For this review, take the finished solid that the model builds, in its own axes (mm). Face numbers are marked on the shaded views. Round coordinates to 2 decimals unless told otherwise and drop trailing zeros. Order: outer loops, then holes, each group sorted by start corner. A loop starts at its lowest first (then second) coordinate and runs counter-clockwise, first axis right, second up.
Autodesk Inventor part; units mm, degrees
ref_plane "YZ Plane" through (0, 0, 0) normal (1, 0, 0) x (0, 1, 0)
ref_plane "XZ Plane" through (0, 0, 0) normal (0, 1, 0) x (-1, 0, 0)
ref_plane "XY Plane" through (0, 0, 0) normal (0, 0, 1) x (1, 0, 0)
sketch "Sketch1" plane through (0, 0, 0) normal (0, 1, 0) x (-1, 0, 0)
  line L0 (0, 0) -> (0, -25.4)
  line L1 (0, -25.4) -> (558.8, -25.4)
  line L2 (558.8, -25.4) -> (558.8, 0)
  line L3 (558.8, 0) -> (0, 0)
  dimension "d0" = 25.4
  dimension "d1" = 558.8
extrude "Plate1" add sketch "Sketch1" along normal blind 0.9652
sketch "Sketch2" plane through (-558.8, 0.1746, -0.5536) normal (0, 0.819152, 0.5735764) x (-1, 0, 0)
  line L0 (-558.8, 0) -> (0, 0)
  line L1 (0, 0) -> (0, 31.75)
  line L2 (0, 31.75) -> (-558.8, 31.75)
  line L3 (-558.8, 31.75) -> (-558.8, 0)
edge flange "Flange1" height 31.75 angle 35 thickness 0.9652 bend radius 0.9652 thickness toward (0, 0.819152, 0.5735764) relief tear relief width 0.9652 relief depth 0.4826 edges at (-279.4, 0, 0) wall of the first edge with corners at (0, 0.1746, -0.5536) (-558.8, 0.1746, -0.5536) (-558.8, -18.0365, 25.4545) (0, -18.0365, 25.4545)
bend "Bend1"
corner "Corner1"
sketch "Sketch3" plane through (0, -17.2459, 24.9008) normal (0, -0.819152, 0.5735764) x (1, 0, 0)
  line L0 (-558.8, 0) -> (0, 0)
  line L1 (0, 0) -> (0, 31.75)
  line L2 (0, 31.75) -> (-558.8, 31.75)
  line L3 (-558.8, 31.75) -> (-558.8, 0)
edge flange "Flange2" height 31.75 angle 70 thickness 0.9652 bend radius 0.9652 thickness toward (0, -0.819152, 0.5735764) relief tear relief width 0.9652 relief depth 0.4826 edges at (-279.4, -17.2459, 26.0081) wall of the first edge with corners at (-558.8, -17.2459, 24.9008) (0, -17.2459, 24.9008) (0, 0.9652, 50.9089) (-558.8, 0.9652, 50.9089)
bend "Bend2"
corner "Corner2"
sketch "Sketch4" plane through (-558.8, 0, 50.9089) normal (0, 1, 0) x (-1, 0, 0)
  line L0 (-558.8, 0) -> (0, 0)
  line L1 (0, 0) -> (0, 25.4)
  line L2 (0, 25.4) -> (-558.8, 25.4)
  line L3 (-558.8, 25.4) -> (-558.8, 0)
edge flange "Flange3" height 25.4 angle 35 thickness 0.9652 bend radius 0.9652 thickness toward (0, 1, 0) relief tear relief width 0.9652 relief depth 0.4826 edges at (-279.4, 0.1746, 51.4625) wall of the first edge with corners at (0, 0, 50.9089) (-558.8, 0, 50.9089) (-558.8, 0, 76.3089) (0, 0, 76.3089)
bend "Bend3"
corner "Corner3"
sketch "Sketch5" plane through (0, 0.9652, 0) normal (0, 1, 0) x (1, 0, 0)
  line L0 (0, -51.5176) -> (-25.4, -51.5176)
  line L1 (0, -51.5176) -> (0, -50.4103)
  line L2 (0, -51.5176) -> (0, 0.6087)
  line L3 (0, 0.6087) -> (-25.4, 0.6087)
  line L4 (-25.4, 0.6087) -> (-25.4, -51.5176)
  line L5 (-114.3, -65.0679) -> (-88.9, -65.0679) construction
  line L6 (-114.3, -67.6079) -> (-88.9, -67.6079)
  line L7 (-88.9, -62.5279) -> (-114.3, -62.5279)
  arc A0 (-114.3, -62.5279) -> (-114.3, -67.6079) centre (-114.3, -65.0679) ccw
  arc A1 (-88.9, -67.6079) -> (-88.9, -62.5279) centre (-88.9, -65.0679) ccw
  line L8 (-87.7062, -24.2598) -> (31.8104, -24.2598) construction
  line L9 (-114.3, 19.0882) -> (-88.9, 19.0882)
  line L10 (-88.9, 14.0082) -> (-114.3, 14.0082)
  arc A2 (-114.3, 19.0882) -> (-114.3, 14.0082) centre (-114.3, 16.5482) ccw
  arc A3 (-88.9, 14.0082) -> (-88.9, 19.0882) centre (-88.9, 16.5482) ccw
  line L11 (0, -76.3089) -> (-558.8, -76.3089)
  line L12 (-279.4, -268.3812) -> (-279.4, 122.1946) construction
  line L13 (-558.8, -51.5176) -> (-533.4, -51.5176)
  line L14 (-558.8, -51.5176) -> (-558.8, 0.6087)
  line L15 (-558.8, 0.6087) -> (-533.4, 0.6087)
  line L16 (-533.4, 0.6087) -> (-533.4, -51.5176)
  line L17 (-444.5, -67.6079) -> (-469.9, -67.6079)
  line L18 (-469.9, -62.5279) -> (-444.5, -62.5279)
  arc A4 (-444.5, -67.6079) -> (-444.5, -62.5279) centre (-444.5, -65.0679) ccw
  arc A5 (-469.9, -62.5279) -> (-469.9, -67.6079) centre (-469.9, -65.0679) ccw
  line L19 (-469.9, 14.0082) -> (-444.5, 14.0082)
  arc A6 (-444.5, 14.0082) -> (-444.5, 19.0882) centre (-444.5, 16.5482) ccw
  line L20 (-444.5, 19.0882) -> (-469.9, 19.0882)
  arc A7 (-469.9, 19.0882) -> (-469.9, 14.0082) centre (-469.9, 16.5482) ccw
  line L21 (0, -51.5176) -> (0, -76.3089)
  point P0 (0, 0)
  point P1 (-101.6, -65.0679)
  point P2 (-457.2, -65.0679)
  dimension "d36" = 25.4
  dimension "d37" = 25.4
  dimension "d38" = 5.08
  dimension "d41" = 88.9
extrude "Cut1" cut sketch "Sketch5" against normal up to next
fillet "Corner Round1" radius 6.35 4 edges at (0, 0.4826, -25.4) (-558.8, 0.4826, 76.3089) (-558.8, 0.4826, -25.4) (0, 0.4826, 76.3089)
fillet "Corner Round2" radius 3.81 4 edges at (-558.8, 0.4826, 51.5176) (0, 0.4826, -0.6087) (0, 0.4826, 51.5176) (-558.8, 0.4826, -0.6087)
sketch "Sketch6" plane through (-533.4, 0.9652, 51.5176) normal (0, 1, 0) x (1, 0, 0)
  point P0 (533.4, 51.5176)
equation "\"d39\" = Thickness"
equation "\"d3\" = BendReliefWidth"
equation "\"d4\" = BendReliefDepth"
equation "\"d5\" = MinimumRemnant"
equation "\"d6\" = BendRadius"
equation "\"d9\" = BendRadius"
equation "\"d10\" = CornerReliefSize"
equation "\"d11\" = GapSize"
equation "\"d12\" = JacobiRadiusSize"
equation "\"d13\" = BendReliefWidth"
equation "\"d14\" = BendReliefDepth"
equation "\"d15\" = MinimumRemnant"
equation "\"d16\" = BendRadius"
equation "\"d19\" = BendRadius"
equation "\"d20\" = CornerReliefSize"
equation "\"d21\" = GapSize"
equation "\"d22\" = JacobiRadiusSize"
equation "\"d23\" = BendReliefWidth"
equation "\"d24\" = BendReliefDepth"
equation "\"d25\" = MinimumRemnant"
equation "\"d26\" = BendRadius"
equation "\"d29\" = BendRadius"
equation "\"d30\" = CornerReliefSize"
equation "\"d31\" = GapSize"
equation "\"d32\" = JacobiRadiusSize"
equation "\"BendRadius\" = Thickness"
equation "\"BendReliefWidth\" = Thickness"
equation "\"BendReliefDepth\" = 0.5 * Thickness"
equation "\"CornerReliefSize\" = 4 * Thickness"
equation "\"MinimumRemnant\" = 2 * Thickness"
equation "\"TransitionRadius\" = BendRadius"
equation "\"JacobiRadiusSize\" = BendRadius"
equation "\"GapSize\" = Thickness"
equation "\"d2\" = BendRadius"
properties part number "Control pipe holder V2" material "Stainless Steel"
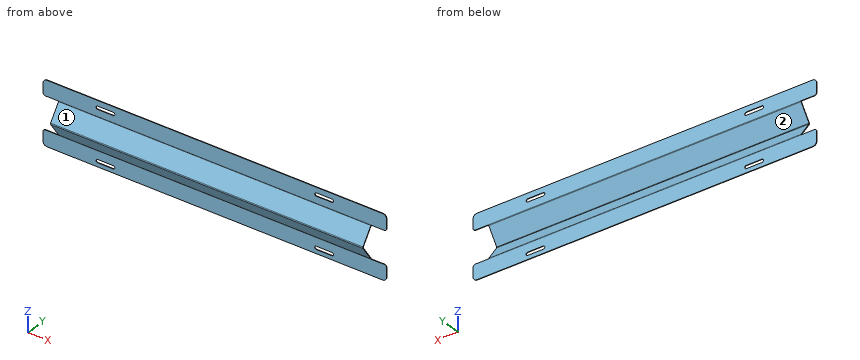
Q1. Mouldability with a two-part tool opening along Z and no side actions: class the marked faces 1 and 2 as +Z half, -Z half, draft (parallel to the pull), parting line (faces both ways), or undercut.
Q2. Wall thickness on line 1 (Y direction, x = -354, z = -14); line 2 (Z direction, x = -44, y = -6.75); line 3 (Z direction, x = -199.5, y = -11.25): over which ranges is each line inside the solid? List them lowest first.
Q3. Take a section at C-C, the plane z = 9.5. State the section outline as (x, y) points, plus the area to 3 significant figures.
Q4. Clearance check with flat-ended pins moving along their axes: pin 1 (2 mm diameter, centred on x = -164.5, y = -12, fed in from +Z); pin 2 (12.5 mm diameter, centred on x = -236, z = -9.5, fed in from -Y); pin 3 (4 mm diameter, centred on x = -176, y = -4.5, fed in from +Z). State where each tip first meets the part, or that it passes through.
Q5. Take a section at A-A, the plane y = -6.5. State the section outline as (x, z) points.
Q6. Take a section at B-B, the plane x = -245.5. State the section outline as (y, z) points.
Working result:
1. face 1: +Z half
1. face 2: undercut
2. line 1: y = 0 to 0.97
2. line 2: z = 9.34 to 11.02, 39.89 to 41.57
2. line 3: z = 15.76 to 17.45, 33.46 to 35.15
3. outline: (-533.4, -6.87) - (-25.4, -6.87) - (-25.4, -5.69) - (-533.4, -5.69) - close
3. area: 599 mm2
4. pin 1: stops at z = 35.5
4. pin 2: stops at y = 0
4. pin 3: stops at z = 47.64
5. outline: (-533.4, 8.98) - (-25.4, 8.98) - (-25.4, 10.66) - (-533.4, 10.66) - close; (-533.4, 40.25) - (-25.4, 40.25) - (-25.4, 41.93) - (-533.4, 41.93) - close
6. outline: (-17.26, 24.35) - (-0.17, -0.05) arc R0.97 cw to (0, -0.61) - (0, -25.4) - (0.97, -25.4) - (0.97, -0.61) arc R1.93 ccw to (0.62, 0.5) - (-16.47, 24.9) arc R0.97 cw to (-16.47, 26.01) - (0.62, 50.41) arc R1.93 ccw to (0.97, 51.52) - (0.97, 76.31) - (0, 76.31) - (0, 51.52) arc R0.97 cw to (-0.17, 50.96) - (-17.26, 26.56) arc R1.93 ccw to start
